Part model, mm, in its own coordinate system. A direction names the side the tool comes from. Coordinates: 2 decimals unless noted, no trailing zeros. Write each loop counter-clockwise with the first axis right and the second up, starting at its lowest first coordinate (ties: lowest second). Pieces come first, ordered by that corner, then holes. Notation, with made-up numbers: M 75.5,-15 L 82.5,-15 A20 ccw 82.5,-10 Z; hole C -36.5,34.5 d3. An arc over 180 degrees is marked long. Use a Markdown table: item, result. Add a question column.
Q1. Mould opens along X. For faces 4 (the cylindrical face through (18.704, -72.938, -3.494)), 5 (the flat face through (30.988, -72, -3)), 6 (the flat face through (0, -0.794, -3)) say: released by +X, released by -X, zero draft, split by the parting line, or undercut.
Q2. Slice it at A-A on y = -120.65. Write the cut outline in (x, z) (1 decimal).
Q3. Wall check: L1, parallel to X at y = -21, z = -1.3; L2, parallel to Y at x = 28.5, z = -2.7; L3, parallel to Y at x = 0, z = -2.55 (3 decimals). Give the ranges that are in metal, low to high. Write a range as from..to.
Q4. Slice it at B-B on x = -7. Write the cut outline in (y, z), then the cut area to 3 significant figures.
Q5. Slice it at D-D on z = -4.5. Count the separate pieces of the cut face and the enclosed holes in it, then the cut area to 3 significant figures.
Q6. Slice it at C-C on x = 6.35. Write the cut outline in (y, z) (1 decimal), then the cut area to 3 significant figures.
Q7. Pin check, flat tips, straight feed: pin 1 Ø2 at (x, z) = (-28, -2.5) entering from +Y; pin 2 Ø2.5 at (y, z) = (-6.5, -4) entering from +X; pin 3 Ø1.2 at (x, z) = (29, -3.5) entering from -Y. Stop position of each tip, or through.
Q8. Tool access for faces 1 (the flat face through (-29, -122.238, -3)), 2 (the flat face through (29, -122.238, -3)), 3 (the flat face through (29, -20.638, -3)): list every direction of +Z, -Z, +X, -X, +Y, -Y with a clear straight run to the whole face (end or side of a thin tool).
from build123d import *

# Parameters (mm, degrees)
BOSS_EXTRUDE1_DEPTH             = 4.7625
F_6_CLEARANCE_HOLE1_D           = 4.3053
F_6_CLEARANCE_HOLE1_DEPTH       = 4.7625
F_3_4_0_75_DIAMETER_HOLE1_D     = 19.05
F_3_4_0_75_DIAMETER_HOLE1_DEPTH = 4.7625


with BuildPart() as part:
    # Sketch1 → Boss-Extrude1 (new body)
    with BuildSketch(Plane.XY.offset(-5.842)):
        with BuildLine():
            Line((-20.5105, -128.5875), (-20.5105, -142.08125))
            Line((-20.5105, -142.08125), (20.5105, -142.08125))
            Line((20.5105, -142.08125), (20.5105, -128.5875))
            ThreePointArc((20.5105, -128.5875), (22.370371939, -124.097371939), (26.8605, -122.2375))
            Line((26.8605, -122.2375), (30.988, -122.2375))
            Line((30.988, -122.2375), (30.988, -20.6375))
            Line((30.988, -20.6375), (26.8605, -20.6375))
            ThreePointArc((26.8605, -20.6375), (22.370371939, -18.777628061), (20.5105, -14.2875))
            Line((20.5105, -14.2875), (20.5105, -0.79375))
            Line((20.5105, -0.79375), (-20.5105, -0.79375))
            Line((-20.5105, -0.79375), (-20.5105, -14.2875))
            ThreePointArc((-20.5105, -14.2875), (-22.370371939, -18.777628061), (-26.8605, -20.6375))
            Line((-26.8605, -20.6375), (-30.988, -20.6375))
            Line((-30.988, -20.6375), (-30.988, -122.2375))
            Line((-30.988, -122.2375), (-26.8605, -122.2375))
            ThreePointArc((-26.8605, -122.2375), (-22.370371939, -124.097371939), (-20.5105, -128.5875))
        make_face()
    extrude(amount=BOSS_EXTRUDE1_DEPTH)

    # #6 Clearance Hole1
    with Locations(Plane.XY.offset(-1.0795)):
        with Locations((-14.605, -13.208), (-23.495, -96.8375), (23.495, -96.8375)):
            Hole(F_6_CLEARANCE_HOLE1_D / 2, depth=F_6_CLEARANCE_HOLE1_DEPTH)

    # 3/4 (0.75) Diameter Hole1
    with Locations(Plane.XY.offset(-1.0795)):
        with Locations((-15.24, -60.325), (6.35, -20.32), (11.684, -79.375), (0, -120.65)):
            Hole(F_3_4_0_75_DIAMETER_HOLE1_D / 2, depth=F_3_4_0_75_DIAMETER_HOLE1_DEPTH)


solid = part.part
Recorded:
| question | item | result |
|---|---|---|
| 1 | face 4 | undercut |
| 1 | face 5 | released by +X |
| 1 | face 6 | zero draft |
| 2 | outline | M -31,-5.8 L -9.5,-5.8 L -9.5,-1.1 L -31,-1.1 Z; M 9.5,-5.8 L 31,-5.8 L 31,-1.1 L 9.5,-1.1 Z |
| 3 | L1 | -30.99..-3.15, 15.85..30.99 |
| 3 | L2 | -122.24..-20.64 |
| 3 | L3 | -142.081..-130.175, -111.125..-27.42, -13.22..-0.794 |
| 4 | outline | M -142.08,-5.84 L -127.11,-5.84 L -127.11,-1.08 L -142.08,-1.08 Z; M -114.19,-5.84 L -65.1,-5.84 L -65.1,-1.08 L -114.19,-1.08 Z; M -55.55,-5.84 L -0.79,-5.84 L -0.79,-1.08 L -55.55,-1.08 Z |
| 4 | area | 566 mm² |
| 5 | separate pieces | 1 |
| 5 | enclosed holes | 7 |
| 5 | area | 6,780 mm² |
| 6 | outline | M -142.1,-5.8 L -127.7,-5.8 L -127.7,-1.1 L -142.1,-1.1 Z; M -113.6,-5.8 L -87.3,-5.8 L -87.3,-1.1 L -113.6,-1.1 Z; M -71.5,-5.8 L -29.8,-5.8 L -29.8,-1.1 L -71.5,-1.1 Z; M -10.8,-5.8 L -0.8,-5.8 L -0.8,-1.1 L -10.8,-1.1 Z |
| 6 | area | 439 mm² |
| 7 | pin 1 | y = -20.64 |
| 7 | pin 2 | x = 20.51 |
| 7 | pin 3 | y = -122.24 |
| 8 | face 1 | +Z, -Z, -X, -Y |
| 8 | face 2 | +Z, -Z, +X, -Y |
| 8 | face 3 | +Z, -Z, +X, +Y |
